```python
from build123d import *

# Parameters (mm, degrees)
SKETCH1_W          = 70
SKETCH1_H          = 15
SKETCH1_R          = 2.04
BASE_FLANGE1_DEPTH = 1.21412
SKETCH3_R          = 10.067909511
CUT_EXTRUDE1_DEPTH = 10
CUT_EXTRUDE2_DEPTH = 10


# Sheet-metal steps are written as plain solids
with BuildPart() as part:
    # Sketch1 → Base-Flange1 (new body)
    with BuildSketch(Plane.XY):
        Rectangle(SKETCH1_W, SKETCH1_H)
        with Locations((-25, 0)):
            Circle(SKETCH1_R, mode=Mode.SUBTRACT)
        with Locations((25, 0)):
            Circle(SKETCH1_R, mode=Mode.SUBTRACT)
    extrude(amount=-BASE_FLANGE1_DEPTH)

    # Sketch3 → Cut-Extrude1 (cut)
    with BuildSketch(Plane.XY):
        with Locations((0, -11.728394917)):
            Circle(SKETCH3_R)
    extrude(amount=-CUT_EXTRUDE1_DEPTH, mode=Mode.SUBTRACT)

    # Sketch4 → Cut-Extrude2 (cut)
    with BuildSketch(Plane(origin=(0, 0, -1.21412), x_dir=(-1, 0, 0), z_dir=(0, 0, -1))):
        with BuildLine():
            Line((27.04, 0), (27.04, -7.5))
            Line((27.04, -7.5), (22.96, -7.5))
            Line((22.96, -7.5), (22.96, 0))
            Line((22.96, 0), (22.96, 3.022234101))
            ThreePointArc((22.96, 3.022234101), (24.907398497, 4.969632598), (26.854796994, 3.022234101))
            Line((26.854796994, 3.022234101), (27.04, 0))
        make_face()
        with BuildLine():
            Line((-22.96, 0), (-22.96, -7.5))
            Line((-22.96, -7.5), (-27.04, -7.5))
            Line((-27.04, -7.5), (-27.04, 0))
            Line((-27.04, 0), (-27.04, 3.022234101))
            ThreePointArc((-27.04, 3.022234101), (-25, 5.062234101), (-22.96, 3.022234101))
            Line((-22.96, 3.022234101), (-22.96, 0))
        make_face()
    extrude(amount=-CUT_EXTRUDE2_DEPTH, mode=Mode.SUBTRACT)


solid = part.part
```
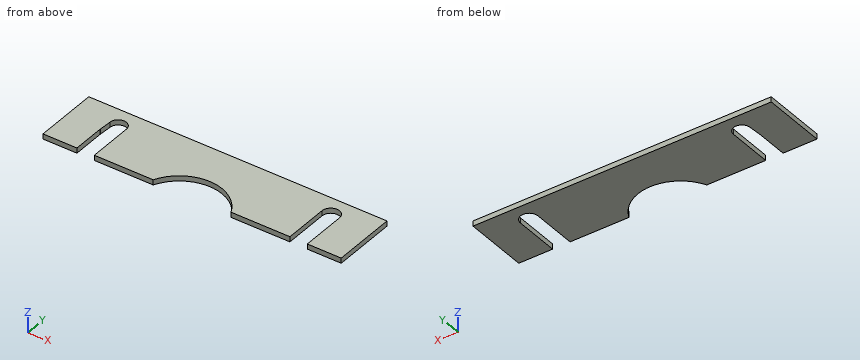
Verification items for the finished model (mm, model axes). Round coordinates to 2 decimals unless told otherwise and drop trailing zeros. Order: outer loops, then holes, each group sorted by start corner. A loop starts at its lowest first (then second) coordinate and runs counter-clockwise, first axis right, second up. Notation, with made-up numbers: (24, -8.75) -> (61, -8.75) arc R31 ccw to (61, 19.25) -> close; hole circle Ø8 at (86, -26). An arc over 180 degrees is marked (long way). Put each result on its own line as item: value. Start each with the question number.
(1) Section check D-D (x = 25). Enter the section's corners in (y, z).
(2) Section check A-A (y = -3). Enter the section's corners in (x, z), then the cut area to 3 significant figures.
(3) Section check C-C (x = 0). Enter the section's corners in (y, z), then the cut area to 3 significant figures.
(4) Material ranges on line 1 along X through (y, z) = (-5, -1); line 2 along X through (y, z) = (3, -0.1); line 3 along X through (y, z) = (0, -0.8), recorded low to high.
(5) Section check B-B (z = -0.3). Enter the section's corners in (x, y), then the cut area to 3 significant figures.
Completed:
1. outline: (5.06, -1.21) -> (7.5, -1.21) -> (7.5, 0) -> (5.06, 0) -> close
2. outline: (-35, -1.21) -> (-27.04, -1.21) -> (-27.04, 0) -> (-35, 0) -> close; (-22.96, -1.21) -> (-5.02, -1.21) -> (-5.02, 0) -> (-22.96, 0) -> close; (5.02, -1.21) -> (22.96, -1.21) -> (22.96, 0) -> (5.02, 0) -> close; (27.04, -1.21) -> (35, -1.21) -> (35, 0) -> (27.04, 0) -> close
2. area: 62.9 mm2
3. outline: (-1.66, -1.21) -> (7.5, -1.21) -> (7.5, 0) -> (-1.66, 0) -> close
3. area: 11.1 mm2
4. line 1: x = -35 to -27.04, -22.96 to -7.49, 7.49 to 22.96, 27.04 to 35
4. line 2: x = -35 to -26.86, -22.96 to 22.96, 27.04 to 35
4. line 3: x = -35 to -27.04, -22.96 to 22.96, 27.04 to 35
5. outline: (-35, -7.5) -> (-27.04, -7.5) -> (-27.04, 0) arc R2.04 cw to (-27.02, 0.25) -> (-26.85, 3.02) arc R1.95 cw to (-22.96, 3.02) -> (-22.96, -7.5) -> (-9.14, -7.5) arc R10.07 cw to (9.14, -7.5) -> (22.96, -7.5) -> (22.96, 3.02) arc R2.04 cw to (27.04, 3.02) -> (27.04, -7.5) -> (35, -7.5) -> (35, 7.5) -> (-35, 7.5) -> close
5. area: 875 mm2
